The model under review builds one solid part; all positions refer to its coordinate system, in mm. A direction names the side the tool comes from. Round coordinates to 2 decimals unless told otherwise and drop trailing zeros. Write each loop counter-clockwise with the first axis right and the second up, starting at its lowest first coordinate (ties: lowest second). Pieces come first, ordered by that corner, then holes. Notation, with made-up numbers: M 19.5,-36 L 32.5,-36 A17 ccw 32.5,-4 Z; hole C 84,59 d5. An arc over 180 degrees is marked long. Write item = value, one per line. Start each with the question number.
Item 1: To check wall thickness, follow line 1 along Y through (x, z) = (6.5, 0); line 2 along Z through (x, y) = (9, 139.2); line 3 along Z through (x, y) = (7.75, 91.5). State the ranges of each line that lie inside material, in increasing order.
Item 2: Take a section at D-D, the plane y = 139.2. Give the boundary of the cut face in (x, z), plus the area to 3 significant figures.
Item 3: For pin 1 Ø3 at (y, z) = (139.2, 5) entering from -X; pin 2 Ø7.5 at (x, y) = (10, 112.5) entering from -Z; pin 3 Ø4.5 at (y, z) = (16.5, 1) entering from -X; pin 4 Ø1 at (x, y) = (6, 41) entering from -Z, all flat-tipped, find the tip position at first contact; note any pin that passes through.
Item 4: Take a section at C-C, the plane x = 2.25. Give the boundary of the cut face in (y, z).
Item 5: Take a section at B-B, the plane z = 0. Give the boundary of the cut face in (x, y).
Item 6: Take a section at A-A, the plane y = 0. Give the boundary of the cut face in (x, z).
Item 7: Tool access review of faces 1 (the cylindrical face through (1.903, -7.496, -0.244)), 2 (the cylindrical face through (7.4, 67.03, -11.67)), 3 (the flat face through (7, 138, 10)), 4 (the flat face through (7, 95, 0)): name each direction out of +Z, -Z, +X, -X, +Y, -Y from which nothing blocks a thin tool from reaching the whole face with its end or side.
Item 8: The part is to be moulded in two halves that separate along Z. For faces 5 (the flat face through (2, 18, 3.5)), 6 (the cylindrical face through (7.395, 89.517, 4.74)), 7 (the cylindrical face through (7.4, 144.27, 8.5)), 8 (the flat face through (7, 135.7, 0)), say which applies: +Z half, -Z half, draft (parallel to the pull), parting line (faces both ways), or undercut.
from build123d import *

# Parameters (mm, degrees)
SKETCH1_R           = 2
BOSS_EXTRUDE1_DEPTH = 15
CUT_EXTRUDE1_DEPTH  = 3.86
SKETCH3_R           = 1.75
CUT_EXTRUDE2_DEPTH  = 148.487591342


with BuildPart() as part:
    # Sketch1 → Boss-Extrude1 (new body)
    with BuildSketch(Plane.YZ):
        with BuildLine():
            Line((95, 10), (40, 10))
            ThreePointArc((40, 10), (22.2375432, 12.29110008), (5.637816862, 19.014424902))
            ThreePointArc((5.637816862, 19.014424902), (4.96102116, 19.331638285), (4.24450028, 19.544416527))
            ThreePointArc((4.24450028, 19.544416527), (-20, 0), (4.24450028, -19.544416527))
            ThreePointArc((4.24450028, -19.544416527), (4.96102116, -19.331638285), (5.637816862, -19.014424902))
            ThreePointArc((5.637816862, -19.014424902), (22.2375432, -12.29110008), (40, -10))
            ThreePointArc((40, -10), (67.41148721, -11.71775609), (94.394082105, -16.844147583))
            ThreePointArc((94.394082105, -16.844147583), (95.008519855, -16.960883889), (95.632724183, -17))
            Line((95.632724183, -17), (140.7, -17))
            ThreePointArc((140.7, -17), (144.235533906, -15.535533906), (145.7, -12))
            Line((145.7, -12), (145.7, 5))
            ThreePointArc((145.7, 5), (144.235533906, 8.535533906), (140.7, 10))
            Line((140.7, 10), (135.7, 10))
            Line((135.7, 10), (135.7, -10))
            Line((135.7, -10), (95, -10))
            Line((95, -10), (95, 10))
        make_face()
        with Locations(Location((139.2, -5, 0), (0, 0, 270))):
            Circle(SKETCH1_R, mode=Mode.SUBTRACT)
        with Locations(Location((139.2, 5, 0), (0, 0, 270))):
            Circle(SKETCH1_R, mode=Mode.SUBTRACT)
        with Locations(Location((91.5, -5, 0), (0, 0, 90))):
            Circle(SKETCH1_R, mode=Mode.SUBTRACT)
        with Locations(Location((91.5, 5, 0), (0, 0, 90))):
            Circle(SKETCH1_R, mode=Mode.SUBTRACT)
    extrude(amount=BOSS_EXTRUDE1_DEPTH)

    # Sketch2 → Cut-Extrude1 (cut)
    with BuildSketch(Plane(origin=(0, 0, 0), x_dir=(0, -1, 0), z_dir=(-1, 0, 0))):
        with BuildLine():
            Line((-24.33053856, -3.5), (-12, -3.5))
            ThreePointArc((-12, -3.5), (-8.440790603, -3.996719292), (-5.153570125, -5.448918697))
            ThreePointArc((-5.153570125, -5.448918697), (7.5, 0), (-5.153570125, 5.448918697))
            ThreePointArc((-5.153570125, 5.448918697), (-8.440790603, 3.996719292), (-12, 3.5))
            Line((-12, 3.5), (-24.33053856, 3.5))
            ThreePointArc((-24.33053856, 3.5), (-27.83053856, 0), (-24.33053856, -3.5))
        make_face()
    extrude(amount=-CUT_EXTRUDE1_DEPTH, mode=Mode.SUBTRACT)

    # Sketch3 → Cut-Extrude2 (cut, through all)
    with BuildSketch(Plane(origin=(3.86, 0, 0), x_dir=(0, -1, 0), z_dir=(-1, 0, 0))):
        with Locations(Location((0, 0, 0), (0, 0, 90))):
            Circle(SKETCH3_R)
        with Locations(Location((-20, 0, 0), (0, 0, 90))):
            Circle(SKETCH3_R)
        with Locations(Location((-24, 0, 0), (0, 0, 90))):
            Circle(SKETCH3_R)
    extrude(amount=-CUT_EXTRUDE2_DEPTH, mode=Mode.SUBTRACT)


solid = part.part
Response values:
q1.line_1 = -20 to -1.75, 1.75 to 18.25, 21.75 to 22.25, 25.75 to 95, 135.7 to 145.7
q1.line_2 = -17 to -7, -3 to 3, 7 to 10
q1.line_3 = -16.13 to -7, -3 to 3, 7 to 10
q2.outline = M 0,-17 L 15,-17 L 15,-7 L 0,-7 Z; M 0,-3 L 15,-3 L 15,3 L 0,3 Z; M 0,7 L 15,7 L 15,10 L 0,10 Z
q2.area = 285 mm2
q3.pin_1 = through
q3.pin_2 = -17
q3.pin_3 = 3.86
q3.pin_4 = -10.01
q4.outline = M 4.24,-19.54 A5 ccw 5.64,-19.01 A70 cw 40,-10 A219.57 cw 94.39,-16.84 A5 ccw 95.63,-17 L 140.7,-17 A5 ccw 145.7,-12 L 145.7,5 A5 ccw 140.7,10 L 135.7,10 L 135.7,-10 L 95,-10 L 95,10 L 40,10 A70 cw 5.64,19.01 A5 ccw 4.24,19.54 A20 ccw long Z; hole M 5.15,-5.45 A13 cw 12,-3.5 L 24.33,-3.5 A3.5 ccw 24.33,3.5 L 12,3.5 A13 cw 5.15,5.45 A7.5 ccw long Z; hole C 91.5,-5 d4; hole C 91.5,5 d4; hole C 139.2,-5 d4; hole C 139.2,5 d4
q5.outline = M 0,-20 L 15,-20 L 15,-1.75 L 3.86,-1.75 L 3.86,-7.5 L 0,-7.5 Z; M 0,27.83 L 3.86,27.83 L 3.86,25.75 L 15,25.75 L 15,95 L 0,95 Z; M 0,135.7 L 15,135.7 L 15,145.7 L 0,145.7 Z; M 3.86,1.75 L 15,1.75 L 15,18.25 L 3.86,18.25 Z; M 3.86,21.75 L 15,21.75 L 15,22.25 L 3.86,22.25 Z
q6.outline = M 0,-20 L 15,-20 L 15,-1.75 L 3.86,-1.75 L 3.86,-7.5 L 0,-7.5 Z; M 0,7.5 L 3.86,7.5 L 3.86,1.75 L 15,1.75 L 15,20 L 0,20 Z
q7.face_1 = -X
q7.face_2 = -Z, +X, -X
q7.face_3 = +Z, +X, -X, +Y
q7.face_4 = +Z, +X, -X
q8.face_5 = undercut
q8.face_6 = undercut
q8.face_7 = +Z half
q8.face_8 = draft
